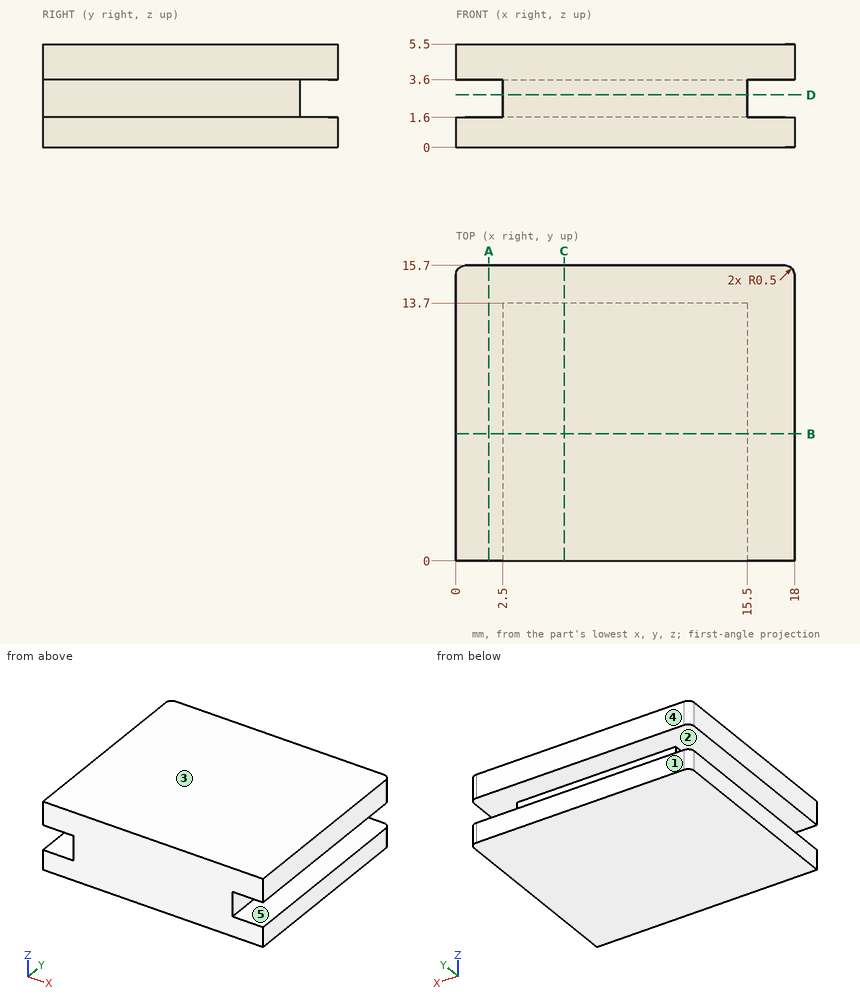
The figure shows three views and two pictorial views of one solid part (mm, origin at its lowest corner). Answer the questions. A direction names the side the tool comes from. Give positions to 0.01 mm unless a question says otherwise; leave off trailing zeros. Loops run counter-clockwise (first coordinate to the right, second up) from the corner with the lowest first, then second, coordinate; pieces in that order, holes last. Notation, with made-up numbers: (28, 2.25) - (37, 2.25) arc R23 ccw to (37, 16.25) - close; hole circle Ø1 at (-15, 10.25). An arc over 180 degrees is marked (long way). Use one line per item in the form item = value.
1. Find the intervals of material crossed by line 1 along Z through (x, y) = (16.75, 15); line 2 along X through (y, z) = (9.5, 2.85); line 3 along Y through (x, z) = (14, 2.95), in increasing order. Write a range as [from, to].
Calculated:
line_1 = [0, 1.6], [3.6, 5.5]
line_2 = [2.5, 15.5]
line_3 = [0, 13.7]
2. Given pin 1 Ø0.6 at (y, z) = (3.5, 2.5) entering from -X; pin 2 Ø0.6 at (x, z) = (11.5, 2.5) entering from +Y, each flat-ended and moving along its own axis, determine where each tip first touches the part or whether it passes through.
Calculated:
pin_1 = 2.5
pin_2 = 13.7
3. Section C-C on x = 5.75 is taken. Give the vertices of the cut face in (y, z), then the cut area to 4 significant figures.
Calculated:
outline = (0, 0) - (15.7, 0) - (15.7, 1.6) - (13.7, 1.6) - (13.7, 3.6) - (15.7, 3.6) - (15.7, 5.5) - (0, 5.5) - close
area = 82.35 mm^2
4. The mould has two halves that part along Z. Classify the marked faces 1, 2 and 3: pulls with the +Z half, pulls with the -Z half, needs draft (parallel to the pull), parting line crosses it, or undercut.
Calculated:
face_1 = needs draft
face_2 = undercut
face_3 = pulls with the +Z half
5. Section D-D on z = 2.8 is taken. Give the vertices of the cut face in (x, y).
Calculated:
outline = (2.5, 0) - (15.5, 0) - (15.5, 13.7) - (2.5, 13.7) - close
6. Section A-A on x = 1.75 is taken. Give the vertices of the cut face in (y, z), then the cut area to 4 significant figures.
Calculated:
outline = (0, 0) - (15.7, 0) - (15.7, 1.6) - (0, 1.6) - close; (0, 3.6) - (15.7, 3.6) - (15.7, 5.5) - (0, 5.5) - close
area = 54.95 mm^2
7. Section B-B on y = 6.75 is taken. Give the vertices of the cut face in (x, z), then the cut area to 3 significant figures.
Calculated:
outline = (0, 0) - (18, 0) - (18, 1.6) - (15.5, 1.6) - (15.5, 3.6) - (18, 3.6) - (18, 5.5) - (0, 5.5) - (0, 3.6) - (2.5, 3.6) - (2.5, 1.6) - (0, 1.6) - close
area = 89.0 mm^2
8. Which of the six approach directions +Z, -Z, +X, -X, +Y, -Y give full straight-line access (tool end or side, diameter ignored) to the marked faces 4 and 5?
Calculated:
face_4 = +Z, -Z, +X, -X, +Y
face_5 = +Y
